Read the model definition and answer for the solid it produces. Units are mm, in the model's axes. Coordinates: 2 decimals unless noted, no trailing zeros. Write each loop counter-clockwise with the first axis right and the second up, starting at its lowest first coordinate (ties: lowest second). Pieces come first, ordered by that corner, then holes. Notation, with made-up numbers: (29, 82.25) -> (73, 82.25) arc R29 ccw to (73, 108.25) -> close; hole circle Ø2 at (64, -4). An arc over 180 degrees is marked (long way). Answer in a Markdown table with one row per item. Add a question column.
Item 1: For a pull along X with two mould halves and no side action, classify faces 1 (the face through (-35, 33.355, 1)), 2 (the face through (-18.106, -99.194, 1.479)), 3 (the face through (-86.065, -39.753, 1.479)), 4 (the face through (-16.6, 10.4, 1.5)) as +X half, -X half, draft (parallel to the pull), parting line (faces both ways), or undercut.
Item 2: Straight lines are drawn through the part: line 1 (Y direction, x = -17, z = 2.2); line 2 (Y direction, x = -44, z = 1.3); line 3 (Y direction, x = -45, z = 2). For each, find the intervals that lie inside material, in ascending order. Write a range as from..to.
Item 3: Section B-B on z = 2.3 is taken. Write down the section's boundary in (x, y).
Item 4: Section D-D on x = -74 is taken. Write down the section's boundary in (y, z), then the cut area to 3 significant figures.
Item 5: Section C-C on x = -57 is taken. Write down the section's boundary in (y, z), then the cut area to 3 significant figures.
Item 6: Section A-A on x = -45 is taken. Write down the section's boundary in (y, z).
```python
from build123d import *
from OCP.BRepFilletAPI import BRepFilletAPI_MakeChamfer

# Parameters (mm, degrees)
SKETCH1_R           = 1.6
SKETCH1_R_2         = 1.5
BOSS_EXTRUDE1_DEPTH = 3
CHAMFER1_SIZE       = 10
CHAMFER1_SIZE2      = 10.020818191
CHAMFER1_SIZE2_2    = 10.605077774


with BuildPart() as part:
    # Sketch1 → Boss-Extrude1 (new body)
    with BuildSketch(Plane.XY):
        Polygon((-82, 33.355339059), (3, 33.355339059), (3, -115.896085726), (-90, -110.53173818), align=None)
        with Locations((-45, 10.355339059)):
            Circle(SKETCH1_R, mode=Mode.SUBTRACT)
        with Locations((-15, 10.355339059)):
            Circle(SKETCH1_R, mode=Mode.SUBTRACT)
        with Locations((-17, -80.208152802)):
            Circle(SKETCH1_R_2, mode=Mode.SUBTRACT)
        with Locations((-17, -100.208152802)):
            Circle(SKETCH1_R_2, mode=Mode.SUBTRACT)
    extrude(amount=BOSS_EXTRUDE1_DEPTH)

    # Chamfer1: one chamfer whose edges measure the first distance from different faces: ONE call of the kernel's chamfer builder (chamfer() names one face for all edges)
    chamfer1_edges_1 = [part.edges().sort_by_distance(p)[0] for p in [
        (-90, -110.53173818, 1.5),
    ]]
    chamfer1_side_1 = [part.faces().sort_by_distance(p)[0] for p in [
        (-86, -38.588199561, 1.5),
    ]]
    chamfer1_edges_2 = [part.edges().sort_by_distance(p)[0] for p in [
        (-82, 33.355339059, 1.5),
    ]]
    chamfer1_side_2 = [part.faces().sort_by_distance(p)[0] for p in [
        (-39.5, 33.355339059, 1.5),
    ]]
    chamfer1 = BRepFilletAPI_MakeChamfer(part.part.solid().wrapped)
    for e in chamfer1_edges_1:
        chamfer1.Add(CHAMFER1_SIZE, CHAMFER1_SIZE2, e.wrapped, chamfer1_side_1[0].wrapped)  # the first distance lies on this face
    for e in chamfer1_edges_2:
        chamfer1.Add(CHAMFER1_SIZE, CHAMFER1_SIZE2_2, e.wrapped, chamfer1_side_2[0].wrapped)  # the first distance lies on this face
    add(Compound.cast(chamfer1.Shape()), mode=Mode.REPLACE)


solid = part.part
```
Results below:
| question | item | result |
|---|---|---|
| 1 | face 1 | draft |
| 1 | face 2 | undercut |
| 1 | face 3 | -X half |
| 1 | face 4 | undercut |
| 2 | line 1 | y = -114.74..-101.71, -98.71..-81.71, -78.71..33.36 |
| 2 | line 2 | y = -113.19..9.11, 11.6..33.36 |
| 2 | line 3 | y = -113.13..8.76, 11.96..33.36 |
| 3 | outline | (-89.44, -100.55) -> (-80, -111.11) -> (3, -115.9) -> (3, 33.36) -> (-72, 33.36) -> (-82.59, 22.77) -> close; hole circle Ø3.2 at (-45, 10.36); hole circle Ø3 at (-17, -100.21); hole circle Ø3 at (-17, -80.21); hole circle Ø3.2 at (-15, 10.36) |
| 4 | outline | (-111.45, 0) -> (31.36, 0) -> (31.36, 3) -> (-111.45, 3) -> close |
| 4 | area | 428 mm2 |
| 5 | outline | (-112.44, 0) -> (33.36, 0) -> (33.36, 3) -> (-112.44, 3) -> close |
| 5 | area | 437 mm2 |
| 6 | outline | (-113.13, 0) -> (8.76, 0) -> (8.76, 3) -> (-113.13, 3) -> close; (11.96, 0) -> (33.36, 0) -> (33.36, 3) -> (11.96, 3) -> close |
